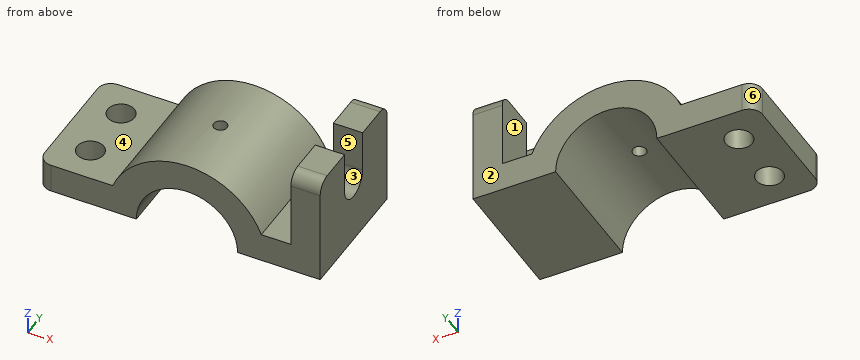
```python
from build123d import *

# Parameters (mm, degrees)
F1_DEPTH  = 48
F2_R      = 5
F3_R      = 5
F5_DEPTH  = 11
F6_R      = 5
F7_R      = 5
F8_R      = 5
F9_DEPTH  = 11
F11_R     = 2.5
F12_DEPTH = 11.1661918982


with BuildPart() as f1:
    # F0 (on Front) → F1 (new body)
    with BuildSketch(Plane.XZ):
        with BuildLine():
            ThreePointArc((-19, 0), (0, 19), (19, 0))
            Line((19, 0), (30, 0))
            Line((30, 0), (50, 0))
            Line((50, 0), (50, 41))
            Line((50, 41), (39, 41))
            Line((39, 41), (39, 11))
            Line((39, 11), (27.9105714739, 11))
            ThreePointArc((27.9105714739, 11), (0, 30), (-27.9105714739, 11))
            Line((-27.9105714739, 11), (-56, 11))
            Line((-56, 11), (-56, 0))
            Line((-56, 0), (-30, 0))
            Line((-30, 0), (-19, 0))
        make_face()
    extrude(amount=F1_DEPTH)

    # F2
    f2_edges = [f1.edges().sort_by_distance(p)[0] for p in [
        (44.5, -48, 41),
    ]]
    fillet(f2_edges, radius=F2_R)

    # F3
    f3_edges = [f1.edges().sort_by_distance(p)[0] for p in [
        (44.5, 0, 41),
    ]]
    fillet(f3_edges, radius=F3_R)

    # F4 (on face) → F5 (cut, through all)
    with BuildSketch(Plane.YZ.offset(50)):
        with BuildLine():
            Line((-17.5, 25), (-17.5, 41))
            Line((-17.5, 41), (-30.5, 41))
            Line((-30.5, 41), (-30.5, 25))
            ThreePointArc((-30.5, 25), (-24, 18.5), (-17.5, 25))
        make_face()
    extrude(amount=-F5_DEPTH, mode=Mode.SUBTRACT)

    # F6
    f6_edges = [f1.edges().sort_by_distance(p)[0] for p in [
        (-56, -48, 5.5),
    ]]
    fillet(f6_edges, radius=F6_R)

    # F7
    f7_edges = [f1.edges().sort_by_distance(p)[0] for p in [
        (-56, 0, 5.5),
    ]]
    fillet(f7_edges, radius=F7_R)

    # F8 (on face) → F9 (cut, through all)
    with BuildSketch(Plane.XY.offset(11)):
        with Locations((-43, -13)):
            Circle(F8_R)
        with Locations((-43, -35)):
            Circle(F8_R)
    extrude(amount=-F9_DEPTH, mode=Mode.SUBTRACT)

    # F11 (on offset) → F12 (cut, through all)
    with BuildSketch(Plane.XY.offset(30)):
        with Locations((0, -24)):
            Circle(F11_R)
    extrude(amount=-F12_DEPTH, mode=Mode.SUBTRACT)


solid = f1.part
```
Geometry check sheet. Reference: the model listing, model coordinates, mm. Face numbers are marked on the shaded views. A direction names the side the tool comes from. Coordinates: 2 decimals unless noted, no trailing zeros. Order: outer loops, then holes, each group sorted by start corner. A loop starts at its lowest first (then second) coordinate and runs counter-clockwise, first axis right, second up.
Item 1: Mould release check, pull along Y, two halves, no side actions. Record for the marked faces 4, 5 and 6: released by +Y, released by -Y, zero draft, split by the parting line, or undercut.
Item 2: Section check B-B (y = -13). Enter the section's corners in (x, z).
Item 3: Section check C-C (z = 21). Enter the section's corners in (x, y), plus the area to 3 significant figures.
Item 4: Tool access check on the marked faces 1, 2 and 3. Record the directions out of +Z, -Z, +X, -X, +Y, -Y that give a thin tool (end or side, any length) a straight path to the whole face; none if there is none.
Item 5: Section check D-D (x = 0). Enter the section's corners in (y, z).
Item 6: Scan lines: line 1 along Y through (x, z) = (-43, 5.25); line 2 along X through (y, z) = (-26, 15.5); line 3 along Y through (x, z) = (0, 25.5). Record each from-to range of solid material in increasing order.
Item 7: Depth check by flat-ended pin: pin 1 (6 mm diameter, centred on x = -40, y = -28.5, fed in from +Z); pin 2 (8 mm diameter, centred on x = 0, y = -24, fed in from +Z); pin 3 (5 mm diameter, centred on x = -21.5, y = -6.5, fed in from +Z); pin 4 (9 mm diameter, centred on x = -43, y = -13, fed in from -Z). Enter the tip coordinate at first touch or a pass-through.
Item 8: Section check A-A (x = -43). Enter the section's corners in (y, z).
Check sheet entries:
1. face 4: zero draft
1. face 5: undercut
1. face 6: released by +Y
2. outline: (-56, 0) - (-48, 0) - (-48, 11) - (-56, 11) - close; (-38, 0) - (-19, 0) arc R19 cw to (19, 0) - (50, 0) - (50, 41) - (39, 41) - (39, 11) - (27.91, 11) arc R30 ccw to (-27.91, 11) - (-38, 11) - close
3. outline: (-21.42, -48) - (21.42, -48) - (21.42, 0) - (-21.42, 0) - close; (39, -48) - (50, -48) - (50, -29.12) - (39, -29.12) - close; (39, -18.88) - (50, -18.88) - (50, 0) - (39, 0) - close; hole circle Ø5 at (0, -24)
3. area: 2,450 mm2
4. face 1: +Z, +Y, -Y
4. face 2: +Z, -Z, +X, -X, +Y
4. face 3: +Z, +X
5. outline: (-48, 19) - (-26.5, 19) - (-26.5, 30) - (-48, 30) - close; (-21.5, 19) - (0, 19) - (0, 30) - (-21.5, 30) - close
6. line 1: y = -48 to -40, -30 to -18, -8 to 0
6. line 2: x = -25.69 to -10.99, 10.99 to 25.69, 39 to 50
6. line 3: y = -48 to -26.5, -21.5 to 0
7. pin 1: stops at z = 11
7. pin 2: stops at z = 30
7. pin 3: stops at z = 23.22
7. pin 4: passes through
8. outline: (-48, 0) - (-40, 0) - (-40, 11) - (-48, 11) - close; (-30, 0) - (-18, 0) - (-18, 11) - (-30, 11) - close; (-8, 0) - (0, 0) - (0, 11) - (-8, 11) - close
